Could you check a few things on this drawing? It's one solid part, dimensions in mm from its lowest x, y, z. A direction names the side the tool comes from. Give positions to 0.01 mm unless a question says otherwise; leave off trailing zeros. Order: outer loops, then holes, each group sorted by start corner. A loop starts at its lowest first (then second) coordinate and runs counter-clockwise, first axis right, second up. Notation, with made-up numbers: (-12, 28) -> (45, 28) arc R24 cw to (45, 47) -> close; hole circle Ø6 at (34.25, 14). An arc over 180 degrees is marked (long way). Answer as a JSON object with one key per item and string values.
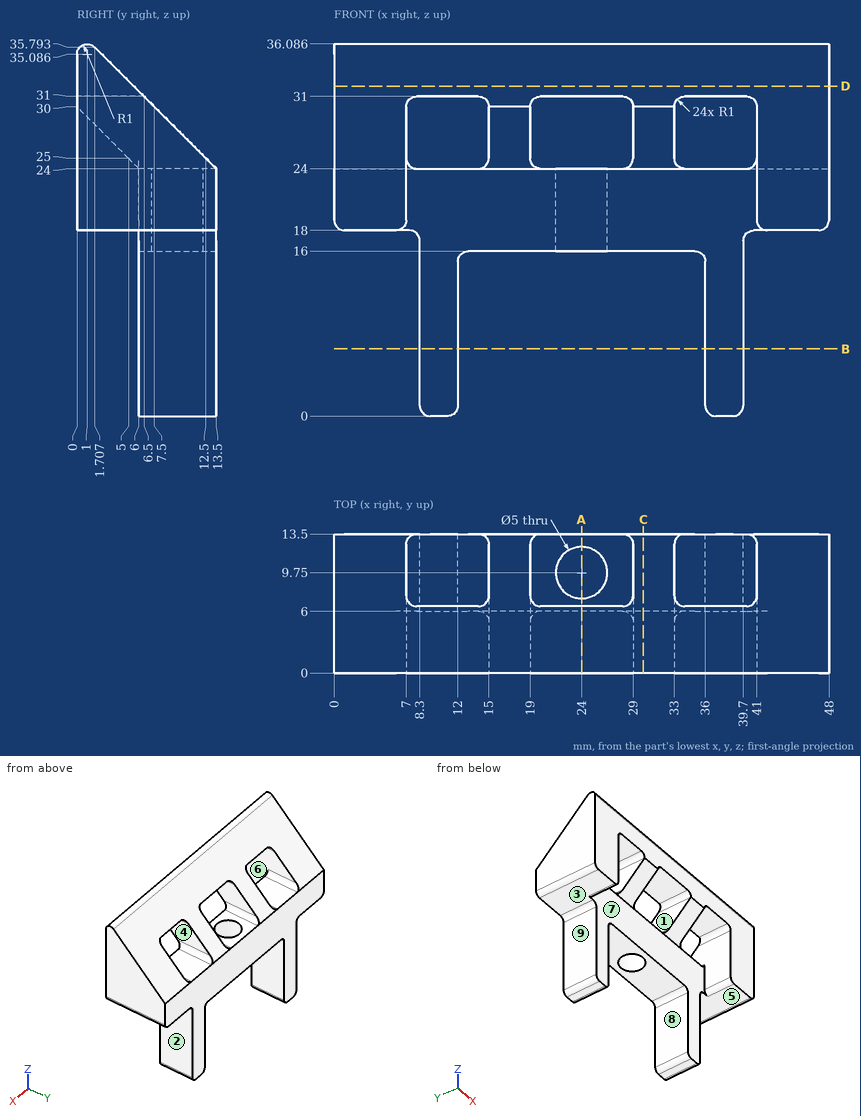
1. If we mould it in two halves opening along Z, with no side actions, what happens to the marked faces 1, 2, 3 and 4? For each: +Z half, -Z half, draft (parallel to the pull), parting line (faces both ways), or undercut.
Worked answers:
{"face 1": "undercut", "face 2": "draft", "face 3": "-Z half", "face 4": "undercut"}
2. If we section it at C-C on x = 30: Please give me the cut outline in (y, z), then the cut area to 3 significant figures.
Worked answers:
{"outline": "(0, 30) -> (6, 24) -> (6, 16) -> (13.5, 16) -> (13.5, 24) -> (1.71, 35.79) arc R1 ccw to (0, 35.09) -> close", "area": "132 mm²"}
3. Will these pins go through, and if not, where does the flat tip stop? pin 1 Ø1.5 at (y, z) = (7.5, 14.5) entering from -X; pin 2 Ø1.9 at (x, y) = (4, 6.5) entering from -Z; pin 3 Ø1 at (x, y) = (23, 5.5) entering from +Z.
Worked answers:
{"pin 1": "x = 8.3", "pin 2": "z = 18", "pin 3": "z = 32.5"}
4. If we section it at B-B on z = 6.5: Please give me the cut outline in (x, y), then the cut area to 3 significant figures.
Worked answers:
{"outline": "(8.3, 6) -> (12, 6) -> (12, 13.5) -> (8.3, 13.5) -> close; (36, 6) -> (39.7, 6) -> (39.7, 13.5) -> (36, 13.5) -> close", "area": "55.5 mm²"}
5. If we section it at A-A on x = 24: Please give me the cut outline in (y, z).
Worked answers:
{"outline": "(0, 31) -> (6.5, 31) -> (1.71, 35.79) arc R1 ccw to (0, 35.09) -> close; (6, 16) -> (7.25, 16) -> (7.25, 24) -> (6, 24) -> close; (12.25, 16) -> (13.5, 16) -> (13.5, 24) -> (12.25, 24) -> close"}
6. If we section it at D-D on z = 32: Please give me the cut outline in (x, y).
Worked answers:
{"outline": "(0, 0) -> (48, 0) -> (48, 5.5) -> (0, 5.5) -> close"}
7. For the marked faces 5, 6, 7, 8 and 9, which set-ups out of +Z, -Z, +X, -X, +Y, -Y let a thin tool reach every point of the face, with its end or its side?
Worked answers:
{"face 5": "-Z, +X, +Y, -Y", "face 6": "-Y", "face 7": "-Z, -Y", "face 8": "-Z, +Y, -Y", "face 9": "-Z, -X, +Y, -Y"}
8. Please list where these lines run through material, in increasing order: L1, parallel to X at y = 9.5, z = 4; L2, parallel to Y at x = 24, z = 21; L3, parallel to X at y = 1, z = 27.
Worked answers:
{"L1": "8.3 to 12, 36 to 39.7", "L2": "6 to 7.25, 12.25 to 13.5", "L3": "0 to 7, 41 to 48"}
